Geometry check sheet. Reference: the model listing, model coordinates, mm. A direction names the side the tool comes from. Give positions to 0.01 mm unless a question says otherwise; leave off trailing zeros. Order: outer loops, then holes, each group sorted by start corner. A loop starts at its lowest first (then second) coordinate and runs counter-clockwise, first axis right, second up.
```python
from build123d import *

# Parameters (mm, degrees)
F0_W           = 6.223
F0_H           = 19.05
F1_DEPTH       = 6.223
F1_DEPTH_BACK  = 19.177
F0_W_2         = 8.89
F2_DEPTH       = 19.177
F5_D           = 4.953
F5_START       = 0.0127
F5_CSINK_D     = 9.652
F5_CSINK_ANGLE = 90


with BuildPart() as f1:
    # F0 (on Top) → F1 (new body, two sides)
    with BuildSketch(Plane.XY) as f1_sk:
        with Locations((-4.445, 0)):
            Rectangle(F0_W, F0_H)
    extrude(amount=F1_DEPTH)
    extrude(f1_sk.sketch, amount=-F1_DEPTH_BACK)

    # F0 (on Top) → F2 (join)
    with BuildSketch(Plane.XY):
        with Locations((3.1115, 0)):
            Rectangle(F0_W_2, F0_H)
        with Locations((-4.445, 0)):
            Rectangle(F0_W, F0_H)
    extrude(amount=-F2_DEPTH)

    # F5 (through all)
    # its depths count from where the whole tool has entered the part; down to there all is cleared
    with Locations(Plane(origin=(-7.5692, 0, 0), x_dir=(0, 1, 0), z_dir=(-1, 0, 0)).offset(-F5_START)):
        with Locations((0, 10.0012505427)):
            CounterSinkHole(F5_D / 2, F5_CSINK_D / 2, counter_sink_angle=F5_CSINK_ANGLE)


solid = f1.part
```
Q1. Cross-section at A-A, the plane y = 0. Record the boundary of the cut face in (x, z).
Q2. Cross-section at C-C, the plane x = 3.5. Record the boundary of the cut face in (y, z) (1 decimal), and give its area (3 significant figures).
Q3. Cross-section at D-D, the plane x = -1.75. Record the boundary of the cut face in (y, z) (1 decimal), and give its area (3 significant figures).
Q4. Thickness scan on L1, parallel to Z at x = 0.75, y = 0; L2, parallel to Y at x = -4, z = -10 (1 decimal); L3, parallel to Z at x = 1.25, y = 4.75. Record the ranges inside material, lowest first.
Q5. Access from +Z, -Z, +X, -X, +Y, -Y to the whole of each face (thin tool, end or side, straight path). Record for faces 1 (the face through (-4, 0, 6.223)), 2 (the face through (-1.334, 0, 3)).
Q6. Cross-section at B-B, the plane y = -6.75. Record the boundary of the cut face in (x, z), and give its area (3 significant figures).
Q7. Gauge pin test, flat ends, axial feed: P1, Ø1, axis at y = -3, z = -9.5, coming from the -X side; P2, Ø7, axis at y = -2, z = 2, coming from the +X side; P3, Ø2.5, axis at x = 4, y = 1.5, coming from the +Z side. Record the tip position at first contact, or that the pin passes through.
Answers follow:
1. outline: (-7.56, -19.18) - (7.56, -19.18) - (7.56, -12.48) - (-5.21, -12.48) - (-7.56, -14.83) - close; (-7.56, -5.18) - (-5.21, -7.52) - (7.56, -7.52) - (7.56, 0) - (-1.33, 0) - (-1.33, 6.22) - (-7.56, 6.22) - close
2. outline: (-9.5, -19.2) - (9.5, -19.2) - (9.5, 0) - (-9.5, 0) - close; hole circle Ø5 at (0, -10)
2. area: 346 mm2
3. outline: (-9.5, -19.2) - (9.5, -19.2) - (9.5, 6.2) - (-9.5, 6.2) - close; hole circle Ø5 at (0, -10)
3. area: 465 mm2
4. L1: z = -19.18 to -12.48, -7.52 to 0
4. L2: y = -9.5 to -2.5, 2.5 to 9.5
4. L3: z = -19.18 to 0
5. face 1: +Z, +X, -X, +Y, -Y
5. face 2: +Z, +X, +Y, -Y
6. outline: (-7.56, -19.18) - (7.56, -19.18) - (7.56, 0) - (-1.33, 0) - (-1.33, 6.22) - (-7.56, 6.22) - close
6. area: 329 mm2
7. P1: stops at x = -6.27
7. P2: stops at x = 7.56
7. P3: stops at z = 0
